Check sheet for the modelled part. Datum: model origin and axes. Units: mm. Face numbers are marked on the shaded views. A direction names the side the tool comes from. Round coordinates to 2 decimals unless told otherwise and drop trailing zeros. Write each loop counter-clockwise with the first axis right and the second up, starting at its lowest first coordinate (ties: lowest second). Pieces come first, ordered by that corner, then holes. Notation, with made-up numbers: M 15,-13.5 L 53,-13.5 A13 ccw 53,6.5 Z; hole C 45,-8.5 d6. An arc over 180 degrees is marked long. One line per item, written item: value.
Autodesk Inventor part; units mm, degrees
ref_plane "YZ Plane" through (0, 0, 0) normal (1, 0, 0) x (0, 1, 0)
ref_plane "XZ Plane" through (0, 0, 0) normal (0, 1, 0) x (-1, 0, 0)
ref_plane "XY Plane" through (0, 0, 0) normal (0, 0, 1) x (1, 0, 0)
sketch "Sketch1" plane through (0, 0, 0) normal (0, 1, 0) x (-1, 0, 0)
  line L0 (0, 0) -> (0, -15)
  line L1 (0, -15) -> (-10, -15)
  line L2 (-10, -15) -> (-10, 0)
  line L3 (-10, 0) -> (0, 0)
  dimension "d0" = 15
  dimension "d1" = 10
extrude "Extrusion1" add sketch "Sketch1" along normal blind 22
sketch "Sketch3" plane through (10, 0, -15) normal (0, 0, -1) x (-1, 0, 0)
  line L0 (0, 0) -> (0, 22)
  line L1 (0, 11) -> (5, 11)
  circle A0 centre (5, 11) radius 2.9
  point P0 (10, 0)
  dimension "d9" = 5
  dimension "d10" = 5.8
extrude "Extrusion3" add sketch "Sketch3" along normal blind 8
sketch "Sketch4" plane through (0, 0, 0) normal (0, -1, 0) x (1, 0, 0)
  line L0 (0, 0) -> (0, -6)
  line L1 (0, -15) -> (0, 0)
  line L2 (0, -6) -> (10, -6)
  line L3 (10, -6.8) -> (0, -6.8)
  line L4 (10, -6) -> (10, -4)
  line L5 (10, -4) -> (0, -4)
  dimension "d13" = 6
  dimension "d14" = 2
extrude "Extrusion4" add sketch "Sketch4" along normal blind 10
fillet "Fillet1" radius 3 2 edges at (10, -10, -5) (0, -10, -5)
sketch "Sketch5" plane through (10, 0, -6) normal (0, 0, -1) x (-1, 0, 0)
  line L0 (0, 0) -> (5, 0)
  line L1 (0, 0) -> (10, 0)
  line L2 (5, 0) -> (5, -5)
  circle A0 centre (5, -5) radius 2
  dimension "d18" = 5
  dimension "d19" = 5
  dimension "d20" = 4
extrude "Extrusion5" cut sketch "Sketch5" against normal blind 10
sketch "Sketch6" plane through (0, 0, 0) normal (0, -1, 0) x (1, 0, 0)
  line L0 (10, -6) -> (10, -15)
  line L1 (10, -15) -> (10, -6)
  line L2 (10, -6) -> (0, -6)
  line L3 (0, -6) -> (0, -15)
  line L4 (0, -15) -> (10, -15)
  line L5 (0, 0) -> (10, 0)
  line L6 (10, -4.0095) -> (0, -4.0095)
  line L7 (0, -4.0095) -> (0, 0)
  line L8 (0, 0) -> (10, 0)
  line L9 (10, 0) -> (10, -4.0095)
extrude "Extrusion6" cut sketch "Sketch6" against normal blind 5.5
sketch "Sketch7" plane through (0, 22, 0) normal (0, 0, 1) x (1, 0, 0)
  line L0 (10, -16.5) -> (10, 0)
  line L1 (10, 0) -> (0, 0)
  line L2 (0, 0) -> (0, -16.5)
  line L3 (0, -16.5) -> (10, -16.5)
  line L4 (10, -16.5) -> (10, 0)
  point P0 (0, -22)
extrude "Extrusion7" add sketch "Sketch7" along normal blind 27
sketch "Sketch8" plane through (10, -7, -4) normal (1, 0, 0) x (0, 0, -1)
  line L0 (11, 29) -> (-31, 29)
  line L1 (11, 29) -> (-25.5, 29)
  line L2 (-25.5, 29) -> (-25.5, 18)
  circle A0 centre (-25.5, 18) radius 2.675
  point P0 (-4, 7)
  dimension "d28" = 36.5
  dimension "d29" = 11
  dimension "d30" = 5.35
extrude "Extrusion8" cut sketch "Sketch8" against normal blind 40
sketch "Sketch9" plane through (0, 22, 0) normal (0, 1, 0) x (1, 0, 0)
  line L0 (0, 15) -> (0, -27)
  line L1 (10, 15) -> (10, -27)
  line L2 (0, -23.4243) -> (10, -23.4243)
  line L3 (10, -23.4243) -> (10, -21.4243)
  line L4 (10, -21.4243) -> (0, -21.4243)
  line L5 (0, -21.4243) -> (0, -23.4243)
  point P0 (0, 0)
  point P1 (0, -21.4243)
  dimension "d33" = 2
extrude "Extrusion9" add sketch "Sketch9" along normal blind 15.5
fillet "Fillet3" radius 3 2 edges at (10, 37.5, 22.4243) (0, 37.5, 22.4243)
sketch "Sketch10" plane through (10, 22, 21.4243) normal (0, 0, -1) x (-1, 0, 0)
  line L0 (7, 15.5) -> (3, 15.5)
  line L1 (5, 15.5) -> (5, 10.5)
  circle A0 centre (5, 10.5) radius 2
  point P0 (10, -22)
  dimension "d37" = 5
  dimension "d38" = 4
extrude "Extrusion10" cut sketch "Sketch10" against normal blind 15.5
sketch "Sketch11" plane through (0, 22, 0) normal (0, 1, 0) x (1, 0, 0)
  line L0 (0, 6) -> (10, 6)
  line L1 (0, 4.0095) -> (10, 4.0095)
  line L2 (0, 6) -> (10, 6)
  line L3 (10, 6) -> (10, 4.0095)
  line L4 (10, 4.0095) -> (0, 4.0095)
  line L5 (0, 4.0095) -> (0, 6)
  point P0 (0, 0)
extrude "Extrusion11" add sketch "Sketch11" along normal blind 15.5
fillet "Fillet4" radius 3 2 edges at (10, 37.5, -5.0048) (0, 37.5, -5.0048)
sketch "Sketch12" plane through (10, 22, -6) normal (0, 0, -1) x (-1, 0, 0)
  circle A0 centre (5, 10.5) radius 2
  circle A1 centre (5, 10.5) radius 2
  point P0 (10, -22)
extrude "Extrusion12" cut sketch "Sketch12" against normal blind 10
sketch "Sketch13" plane through (0, 5.5, 0) normal (0, -1, 0) x (1, 0, 0)
  line L0 (10, 18.825) -> (0, 18.825)
  line L1 (0, 21.4243) -> (10, 21.4243)
  line L2 (10, 18.825) -> (0, 18.825)
  line L3 (0, 18.825) -> (0, 21.4243)
  line L4 (0, 21.4243) -> (10, 21.4243)
  line L5 (10, 21.4243) -> (10, 18.825)
  point P0 (0, 0)
extrude "Extrusion13" add sketch "Sketch13" along normal blind 15.5
fillet "Fillet5" radius 3 2 edges at (0, -10, 20.1246) (10, -10, 20.1246)
sketch "Sketch14" plane through (0, 5.5, 21.4243) normal (0, 0, 1) x (1, 0, 0)
  circle A0 centre (5, -10.5) radius 2
  circle A1 centre (5, -10.5) radius 2
  point P0 (0, -5.5)
extrude "Extrusion14" cut sketch "Sketch14" against normal blind 15.5
properties part number "DudukanRodaDepan"
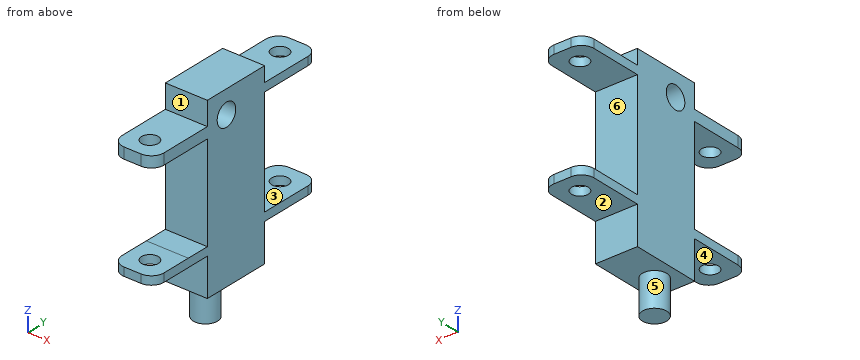
Q1. Draft check along Z on the marked faces 1, 2 and 3. Enter one of: pulls with the +Z half, pulls with the -Z half, needs draft (parallel to the pull), parting line crosses it, or undercut.
Completed:
face 1: needs draft
face 2: pulls with the -Z half
face 3: undercut
Q2. Sectioned sample at C-C on x = 5. State how many separate pieces and enclosed holes the cut face has, and give its area (3 significant figures).
Completed:
separate pieces: 5
enclosed holes: 1
area: 816 mm^2
Q3. Access from +Z, -Z, +X, -X, +Y, -Y to the whole of each face (thin tool, end or side, straight path). Record for the marked faces 4, 5 and 6.
Completed:
face 4: -Z, +X, -X, -Y
face 5: -Z
face 6: +X, -X, +Y
Q4. Depth check by flat-ended pin: P1, Ø5, axis at x = 4, y = 26.5, coming from the -Z side; P2, Ø4, axis at x = 3, y = 17, coming from the -Z side; P3, Ø3, axis at x = 1.5, z = -14, coming from the -Y side. Enter the tip coordinate at first touch or a pass-through.
Completed:
P1: z = -6
P2: z = -15
P3: y = 5.5
Q5. Sectioned sample at A-A on y = 29. Enter the section's corners in (x, z), and give its area (3 significant figures).
Completed:
outline: M 0,-6 L 10,-6 L 10,-4.01 L 0,-4.01 Z; M 0,21.42 L 10,21.42 L 10,23.42 L 0,23.42 Z
area: 39.9 mm^2
Q6. Sectioned sample at B-B on y = -5. Enter the section's corners in (x, z) (3 decimals), and give its area (3 significant figures).
Completed:
outline: M 0,-6 L 3,-6 L 3,-4 L 0,-4 Z; M 0,18.825 L 3,18.825 L 3,21.424 L 0,21.424 Z; M 7,-6 L 10,-6 L 10,-4 L 7,-4 Z; M 7,18.825 L 10,18.825 L 10,21.424 L 7,21.424 Z
area: 27.6 mm^2
Q7. Sectioned sample at D-D on z = 7. Enter the section's corners in (x, y), and give its area (3 significant figures).
Completed:
outline: M 0,5.5 L 10,5.5 L 10,22 L 0,22 Z
area: 165 mm^2
Q8. Scan lines: line 1 (Y direction, x = 5, z = -4.85); line 2 (Z direction, x = 7.5, y = 11) (3 decimals); line 3 (Z direction, x = 1.75, y = 34.5). Record each from-to range of solid material in increasing order. Write a range as [from, to].
Completed:
line 1: [-10, -7], [-3, 30.5], [34.5, 37.5]
line 2: [-23, 18.825], [24.175, 27]
line 3: [-6, -4.01], [21.42, 23.42]
